Model file for the job. Use its own axes, mm. Round coordinates to 2 decimals unless told otherwise and drop trailing zeros. Write each loop counter-clockwise with the first axis right and the second up, starting at its lowest first coordinate (ties: lowest second). Pieces come first, ordered by that corner, then holes.
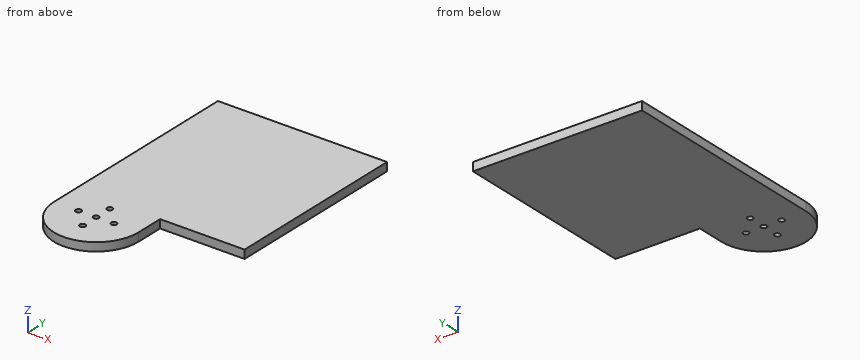
```python
from build123d import *

# Parameters (mm, degrees)
SKETCH_1_R      = 15
SKETCH_1_R_2    = 1
EXTRUDE_1_DEPTH = 3
SKETCH_2_W      = 3
SKETCH_2_H      = 66
EXTRUDE_2_DEPTH = 30


with BuildPart() as part:
    # 草圖1 → 填料-伸長1 (new body)
    with BuildSketch(Plane.XY):
        Circle(SKETCH_1_R)
        with Locations((0, 6.3)):
            Circle(SKETCH_1_R_2, mode=Mode.SUBTRACT)
        with Locations((-6.3, 0)):
            Circle(SKETCH_1_R_2, mode=Mode.SUBTRACT)
        with Locations((0, -6.3)):
            Circle(SKETCH_1_R_2, mode=Mode.SUBTRACT)
        with Locations((6.3, 0)):
            Circle(SKETCH_1_R_2, mode=Mode.SUBTRACT)
        Circle(SKETCH_1_R_2, mode=Mode.SUBTRACT)
        with BuildLine():
            Line((-15, 76), (-15, 0))
            ThreePointArc((-15, 0), (0, 15), (15, 0))
            Line((15, 0), (15, 76))
            Line((15, 76), (-15, 76))
        make_face()
    extrude(amount=-EXTRUDE_1_DEPTH)

    # 草圖2 → 填料-伸長2 (add)
    with BuildSketch(Plane(origin=(15, 0, 0), x_dir=(0, 0, -1), z_dir=(1, 0, 0))):
        with Locations((1.5, 43)):
            Rectangle(SKETCH_2_W, SKETCH_2_H)
    extrude(amount=EXTRUDE_2_DEPTH)


solid = part.part
```
1) Cut at A-A on y = 6.3. List the corners of the cut face in (x, z).
2) Wall check: probe 1 along Y at (x, z) = (0, -2.1); probe 2 along X at (y, z) = (-7, -1.05); probe 3 along Y at (x, z) = (35.5, -0.15). Give the ranges that are in metal, low to high.
3) Cut at C-C on z = -0.95. List the corners of the cut face in (x, y), and give its area (3 significant figures).
4) Cut at B-B on x = 0. List the corners of the cut face in (y, z), and give its area (3 significant figures).
5) Flat gauge pins, fed straight in: pin 1 Ø1.8 at (x, y) = (-6.3, 0) entering from +Z; pin 2 Ø1.5 at (x, z) = (36.5, -1.5) entering from -Y. Where does each tip first touch, or does it go through?
6) Cut at D-D on x = 6.3. List the corners of the cut face in (y, z).
Result sheet:
1. outline: (-15, -3) - (-1, -3) - (-1, 0) - (-15, 0) - close; (1, -3) - (15, -3) - (15, 0) - (1, 0) - close
2. probe 1: y = -15 to -7.3, -5.3 to -1, 1 to 5.3, 7.3 to 76
2. probe 2: x = -13.27 to -0.71, 0.71 to 13.27
2. probe 3: y = 10 to 76
3. outline: (-15, 0) arc R15 ccw to (15, 0) - (15, 10) - (45, 10) - (45, 76) - (-15, 76) - close; hole circle Ø2 at (-6.3, 0); hole circle Ø2 at (0, -6.3); hole circle Ø2 at (0, 0); hole circle Ø2 at (0, 6.3); hole circle Ø2 at (6.3, 0)
3. area: 4,600 mm2
4. outline: (-15, -3) - (-7.3, -3) - (-7.3, 0) - (-15, 0) - close; (-5.3, -3) - (-1, -3) - (-1, 0) - (-5.3, 0) - close; (1, -3) - (5.3, -3) - (5.3, 0) - (1, 0) - close; (7.3, -3) - (76, -3) - (76, 0) - (7.3, 0) - close
4. area: 255 mm2
5. pin 1: passes through
5. pin 2: stops at y = 10
6. outline: (-13.61, -3) - (-1, -3) - (-1, 0) - (-13.61, 0) - close; (1, -3) - (76, -3) - (76, 0) - (1, 0) - close
